from build123d import *

# Parameters (mm, degrees)
BOSS_EXTRUDE6_DEPTH      = 6
BOSS_EXTRUDE7_DEPTH      = 0.995824486
BOSS_EXTRUDE7_DEPTH_BACK = 1.5
FILLET17_R               = 2
SKETCH4_R                = 2.5
CUT_EXTRUDE2_DEPTH       = 11.5
SKETCH11_R               = 1.4
CUT_EXTRUDE3_DEPTH       = 15
CUT_EXTRUDE10_DEPTH      = 0.5
CUT_EXTRUDE10_DEPTH_BACK = 2
SKETCH14_W               = 2.5
SKETCH14_H               = 6.5
CUT_EXTRUDE15_DEPTH      = 8.75
SKETCH16_R               = 1.85
CUT_EXTRUDE16_DEPTH      = 15


with BuildPart() as part:
    # Sketch1 → Boss-Extrude6 (new body)
    with BuildSketch(Plane(origin=(0, 0, 0), x_dir=(1, 0, 0), z_dir=(0, 1, 0))):
        with BuildLine():
            ThreePointArc((12, 0), (8.485281374, 8.485281374), (0, 12))
            ThreePointArc((0, 12), (-8.485281374, 8.485281374), (-12, 0))
            ThreePointArc((-12, 0), (-8.485281374, -8.485281374), (0, -12))
            ThreePointArc((0, -12), (8.485281374, -8.485281374), (12, 0))
        make_face()
    extrude(amount=BOSS_EXTRUDE6_DEPTH)

    # Sketch1<11> → Boss-Extrude7 (add, two sides: drawn at the far end of the back side and taken through both)
    with BuildSketch(Plane(origin=(0, 0, 0), x_dir=(1, 0, 0), z_dir=(0, 1, 0)).offset(-BOSS_EXTRUDE7_DEPTH_BACK)):
        with BuildLine():
            ThreePointArc((15, 0), (10.606601718, 10.606601718), (0, 15))
            ThreePointArc((0, 15), (-10.606601718, 10.606601718), (-15, 0))
            ThreePointArc((-15, 0), (-10.606601718, -10.606601718), (0, -15))
            ThreePointArc((0, -15), (10.606601718, -10.606601718), (15, 0))
        make_face()
        with BuildLine():
            ThreePointArc((12, 0), (8.485281374, 8.485281374), (0, 12))
            ThreePointArc((0, 12), (-8.485281374, 8.485281374), (-12, 0))
            ThreePointArc((-12, 0), (-8.485281374, -8.485281374), (0, -12))
            ThreePointArc((0, -12), (8.485281374, -8.485281374), (12, 0))
        make_face(mode=Mode.SUBTRACT)
    extrude(amount=BOSS_EXTRUDE7_DEPTH + BOSS_EXTRUDE7_DEPTH_BACK)


with BuildPart() as boss_extrude7_kept_piece:
    # of the separate pieces the step leaves, the one the design keeps (boss_extrude7_pieces_kept)
    add(part.part.solids().sort_by_distance((12, 6, 0))[0])

    # Fillet17
    # the kernel refuses this fillet: 2 mm, written as the material it adds along each edge
    with BuildSketch(Plane(origin=(0, 0, 0), x_dir=(1, 0, 0), z_dir=(0, 0, 1))) as fillet17_piece_1:
        with BuildLine():
            CenterArc((10.063508327, -2), FILLET17_R, 14.477512186, 75.522487814)
            Line((10.063508327, 0), (10.063508327, 0.04))
            Line((10.063508327, 0.04), (12, 0.04))
            Line((12, 0.04), (12.04, 0))
            ThreePointArc((12.04, 0), (12.04, -0.75), (12.038729833, -1.49))
            Line((12.038729833, -1.49), (12, -1.5))
        make_face()
    revolve(axis=Axis((0, 0, 0), (0, 1, 0)))

    # Sketch4 → Cut-Extrude2 (cut)
    with BuildSketch(Plane(origin=(0, 6, 0), x_dir=(1, 0, 0), z_dir=(0, 1, 0))):
        with Locations(Location((0, 0, 0), (0, 0, 270))):
            Circle(SKETCH4_R)
    extrude(amount=-CUT_EXTRUDE2_DEPTH, mode=Mode.SUBTRACT)

    # Mirror6: Boss-Extrude7 kept piece across plane


with BuildPart() as boss_extrude7_kept_piece_1:
    add(boss_extrude7_kept_piece.part)
    add(boss_extrude7_kept_piece.part.mirror(Plane.ZX.offset(6)))

    # Sketch11 → Cut-Extrude3 (cut)
    with BuildSketch(Plane(origin=(0, 0, 0), x_dir=(0, 0, -1), z_dir=(1, 0, 0))):
        with Locations((0, 6)):
            Circle(SKETCH11_R)
    extrude(amount=-CUT_EXTRUDE3_DEPTH, mode=Mode.SUBTRACT)

    # Sketch12 → Cut-Extrude10 (cut, two sides: drawn at the far end of the back side and taken through both)
    with BuildSketch(Plane(origin=(-3.5, 0, 0), x_dir=(0, 0, -1), z_dir=(1, 0, 0)).offset(-CUT_EXTRUDE10_DEPTH_BACK)):
        Polygon((3.175426481, 6), (1.58771324, 8.75), (-1.58771324, 8.75), (-3.175426481, 6), (-1.58771324, 3.25), (1.58771324, 3.25), align=None)
    extrude(amount=CUT_EXTRUDE10_DEPTH + CUT_EXTRUDE10_DEPTH_BACK, mode=Mode.SUBTRACT)

    # Sketch14 → Cut-Extrude15 (cut)
    with BuildSketch(Plane.XZ):
        with Locations((-4.75, 0)):
            Rectangle(SKETCH14_W, SKETCH14_H)
    extrude(amount=-CUT_EXTRUDE15_DEPTH, mode=Mode.SUBTRACT)

    # Sketch16 → Cut-Extrude16 (cut)
    with BuildSketch(Plane(origin=(0, 0, 0), x_dir=(0, 0, -1), z_dir=(1, 0, 0))):
        with Locations(Location((0, 6, 0), (0, 0, 180))):
            Circle(SKETCH16_R)
    extrude(amount=CUT_EXTRUDE16_DEPTH, mode=Mode.SUBTRACT)


solid = boss_extrude7_kept_piece_1.part
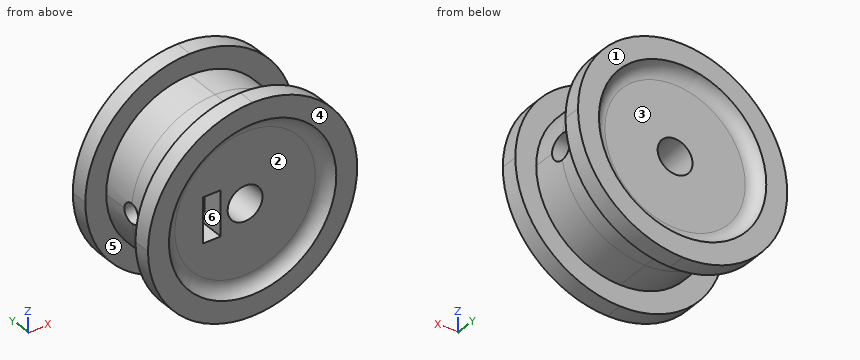
Source: CAD feature listing. Evaluate the final solid. Frame: model axes, mm. Face numbers are marked on the shaded views. A direction names the side the tool comes from. Give positions to 0.01 mm unless a question says otherwise; leave off trailing zeros. Write each loop counter-clockwise with the first axis right and the second up, starting at its lowest first coordinate (ties: lowest second). Pieces come first, ordered by that corner, then holes. Notation, with made-up numbers: M 87,15.25 L 92,15.25 A9 ccw 92,22.25 Z; hole C -5.75,72 d8. An arc over 180 degrees is marked long. Return JSON: item names as keys, results as strings. Group by question number.
1) Cut plane A-A, the plane y = 2.25. Output: boundary loops of the cut face in (x, z), plus the area to 3 significant figures.
2) Pull-direction query (Z, two-part tool) for the marked faces 1 and 2; classes: pulls with the +Z half, pulls with the -Z half, needs draft (parallel to the pull), parting line crosses it, or undercut.
3) Cut plane B-B, the plane y = 5.5. Output: boundary loops of the cut face in (x, z), plus the area to 3 significant figures.
4) Pin query (flat end, axial travel): P1, Ø2, axis at x = -4, y = 2.5, coming from the -Z side; P2, Ø2, axis at x = 4.5, y = 7, coming from the +Z side; P3, Ø3, axis at x = 0, z = -9, coming from the -Y side. Return the tip coordinate at first contact, or that it passes through.
5) Material intervals for line 1 along Y through (x, z) = (-2.8, 0); line 2 along Y through (x, z) = (3.25, 0); line 3 along X through (y, z) = (-0.25, 5.5), sorted ascending. Write a range as [from, to].
6) Set-up query: the marked faces 3, 4, 5 and 6. Return all of +Z, -Z, +X, -X, +Y, -Y with unobstructed straight access to the full face (end or side cutting, diameter ignored); none if empty.
Recorded:
{
 "1": {"outline": "C 0,0 d24; hole M -6,-3.25 L -3.5,-3.25 L -3.5,3.25 L -6,3.25 Z; hole C 0,0 d5", "area": "417 mm²"},
 "2": {"face 1": "needs draft", "face 2": "undercut"},
 "3": {"outline": "M -11.93,-1.31 A12 ccw 11.87,-1.78 L 1.75,-1.78 A2.5 cw -2.13,-1.31 L -3,-1.31 L -3,-2.89 L -3.5,-2.89 L -3.5,-3.25 L -6,-3.25 L -6,-1.31 Z; M -11.93,1.31 L -6,1.31 L -6,3.25 L -3.5,3.25 L -3.5,2.89 L -3,2.89 L -3,1.31 L -2.13,1.31 A2.5 cw 1.75,1.78 L 11.87,1.78 A12 ccw Z", "area": "362 mm²"},
 "4": {"P1": "stops at z = -11.62", "P2": "stops at z = 11.48", "P3": "stops at y = -0.05"},
 "5": {"line 1": "y = [0, 4.6], [7.4, 12]", "line 2": "y = [0, 4.15], [7.85, 12]", "line 3": "x = [-13.96, -9.56], [9.56, 13.96]"},
 "6": {"face 3": "+Y", "face 4": "+Z, -Z, +X, -X, -Y", "face 5": "none", "face 6": "-Y"}
}
